Geometry check sheet. Reference: drawing and pictorial views, mm from the part's lowest x, y, z. Give positions to 0.01 mm unless a question says otherwise; leave off trailing zeros. Write each loop counter-clockwise with the first axis right and the second up, starting at its lowest first coordinate (ties: lowest second). Pieces come first, ordered by that corner, then holes. Notation, with made-up numbers: (50, 66) -> (58, 66) arc R25 cw to (58, 92) -> close; hole circle Ø9 at (38, -29.5). An arc over 180 degrees is marked (long way). Use a Markdown table: item, result. Add a question column.
1. Cross-section at B-B (z = 3.5). Enter the section's corners in (x, y), then the cut area to 3 significant figures.
2. Cross-section at A-A (x = 110.5). Enter the section's corners in (y, z), then the cut area to 3 significant figures.
3. Scan line: probe 1 along Z at (x, y) = (110.5, 1.2). Record every from-to range of solid material in increasing order. Write a range as [from, to].
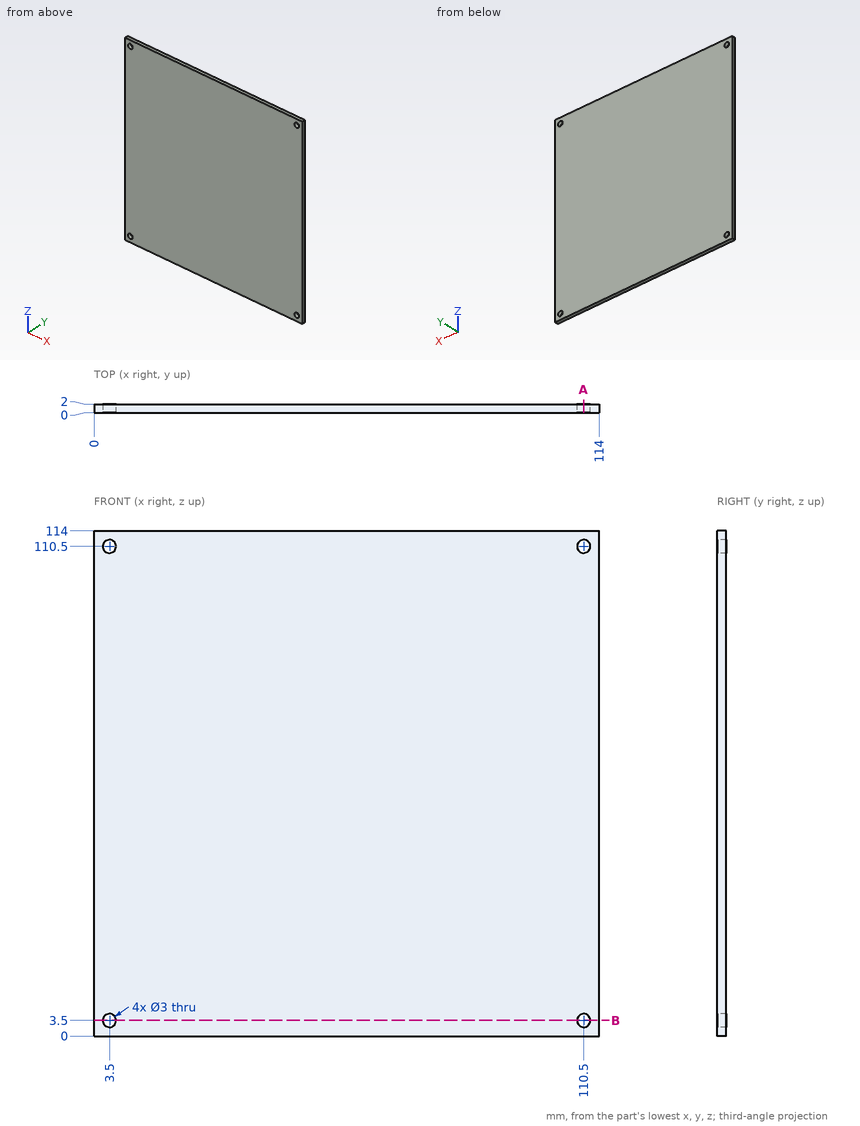
Worked answers:
| question | item | result |
|---|---|---|
| 1 | outline | (0, 0) -> (2, 0) -> (2, 2) -> (0, 2) -> close; (5, 0) -> (109, 0) -> (109, 2) -> (5, 2) -> close; (112, 0) -> (114, 0) -> (114, 2) -> (112, 2) -> close |
| 1 | area | 216 mm² |
| 2 | outline | (0, 0) -> (2, 0) -> (2, 2) -> (0, 2) -> close; (0, 5) -> (2, 5) -> (2, 109) -> (0, 109) -> close; (0, 112) -> (2, 112) -> (2, 114) -> (0, 114) -> close |
| 2 | area | 216 mm² |
| 3 | probe 1 | z = [0, 2], [5, 109], [112, 114] |
